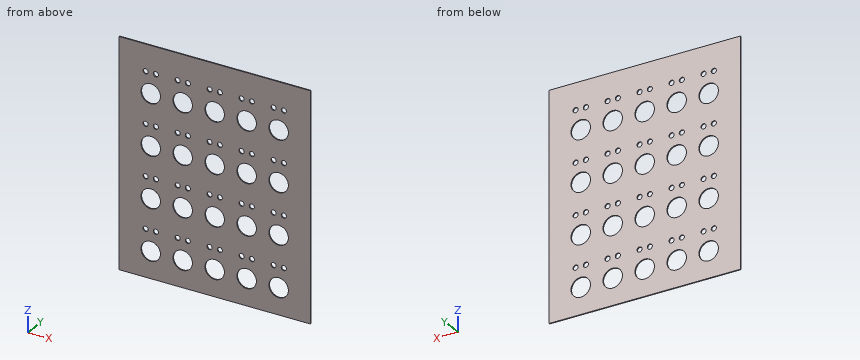
```python
from build123d import *

# Parameters (mm, degrees)
SKETCH1_W           = 187
SKETCH1_H           = 222
SKETCH1_R           = 2.5
SKETCH1_R_2         = 9.5
BOSS_EXTRUDE1_DEPTH = 1


with BuildPart() as part:
    # Sketch1 → Boss-Extrude1 (new body)
    with BuildSketch(Plane(origin=(0, 0, 0), x_dir=(1, 0, 0), z_dir=(0, 1, 0))):
        with Locations((64.462554676, 36.018217652)):
            Rectangle(SKETCH1_W, SKETCH1_H)
        with Locations((-3.037445324, -48.981782348)):
            Circle(SKETCH1_R, mode=Mode.SUBTRACT)
        with Locations((6.962554676, -48.981782348)):
            Circle(SKETCH1_R, mode=Mode.SUBTRACT)
        with Locations((28.212554676, -48.981782348)):
            Circle(SKETCH1_R, mode=Mode.SUBTRACT)
        with Locations((38.212554676, -48.981782348)):
            Circle(SKETCH1_R, mode=Mode.SUBTRACT)
        with Locations((1.962554676, -28.981782348)):
            Circle(SKETCH1_R_2, mode=Mode.SUBTRACT)
        with Locations((33.212554676, -28.981782348)):
            Circle(SKETCH1_R_2, mode=Mode.SUBTRACT)
        with Locations((59.462554676, -48.981782348)):
            Circle(SKETCH1_R, mode=Mode.SUBTRACT)
        with Locations((69.462554676, -48.981782348)):
            Circle(SKETCH1_R, mode=Mode.SUBTRACT)
        with Locations((64.462554676, -28.981782348)):
            Circle(SKETCH1_R_2, mode=Mode.SUBTRACT)
        with Locations((90.712554676, -48.981782348)):
            Circle(SKETCH1_R, mode=Mode.SUBTRACT)
        with Locations((100.712554676, -48.981782348)):
            Circle(SKETCH1_R, mode=Mode.SUBTRACT)
        with Locations((95.712554676, -28.981782348)):
            Circle(SKETCH1_R_2, mode=Mode.SUBTRACT)
        with Locations((121.962554676, -48.981782348)):
            Circle(SKETCH1_R, mode=Mode.SUBTRACT)
        with Locations((131.962554676, -48.981782348)):
            Circle(SKETCH1_R, mode=Mode.SUBTRACT)
        with Locations((126.962554676, -28.981782348)):
            Circle(SKETCH1_R_2, mode=Mode.SUBTRACT)
        with Locations((-3.037445324, 1.018217652)):
            Circle(SKETCH1_R, mode=Mode.SUBTRACT)
        with Locations((6.962554676, 1.018217652)):
            Circle(SKETCH1_R, mode=Mode.SUBTRACT)
        with Locations((1.962554676, 21.018217652)):
            Circle(SKETCH1_R_2, mode=Mode.SUBTRACT)
        with Locations((28.212554676, 1.018217652)):
            Circle(SKETCH1_R, mode=Mode.SUBTRACT)
        with Locations((38.212554676, 1.018217652)):
            Circle(SKETCH1_R, mode=Mode.SUBTRACT)
        with Locations((33.212554676, 21.018217652)):
            Circle(SKETCH1_R_2, mode=Mode.SUBTRACT)
        with Locations((59.462554676, 1.018217652)):
            Circle(SKETCH1_R, mode=Mode.SUBTRACT)
        with Locations((69.462554676, 1.018217652)):
            Circle(SKETCH1_R, mode=Mode.SUBTRACT)
        with Locations((64.462554676, 21.018217652)):
            Circle(SKETCH1_R_2, mode=Mode.SUBTRACT)
        with Locations((90.712554676, 1.018217652)):
            Circle(SKETCH1_R, mode=Mode.SUBTRACT)
        with Locations((100.712554676, 1.018217652)):
            Circle(SKETCH1_R, mode=Mode.SUBTRACT)
        with Locations((95.712554676, 21.018217652)):
            Circle(SKETCH1_R_2, mode=Mode.SUBTRACT)
        with Locations((121.962554676, 1.018217652)):
            Circle(SKETCH1_R, mode=Mode.SUBTRACT)
        with Locations((131.962554676, 1.018217652)):
            Circle(SKETCH1_R, mode=Mode.SUBTRACT)
        with Locations((126.962554676, 21.018217652)):
            Circle(SKETCH1_R_2, mode=Mode.SUBTRACT)
        with Locations((-3.037445324, 51.018217652)):
            Circle(SKETCH1_R, mode=Mode.SUBTRACT)
        with Locations((6.962554676, 51.018217652)):
            Circle(SKETCH1_R, mode=Mode.SUBTRACT)
        with Locations((1.962554676, 71.018217652)):
            Circle(SKETCH1_R_2, mode=Mode.SUBTRACT)
        with Locations((28.212554676, 51.018217652)):
            Circle(SKETCH1_R, mode=Mode.SUBTRACT)
        with Locations((38.212554676, 51.018217652)):
            Circle(SKETCH1_R, mode=Mode.SUBTRACT)
        with Locations((33.212554676, 71.018217652)):
            Circle(SKETCH1_R_2, mode=Mode.SUBTRACT)
        with Locations((59.462554676, 51.018217652)):
            Circle(SKETCH1_R, mode=Mode.SUBTRACT)
        with Locations((69.462554676, 51.018217652)):
            Circle(SKETCH1_R, mode=Mode.SUBTRACT)
        with Locations((64.462554676, 71.018217652)):
            Circle(SKETCH1_R_2, mode=Mode.SUBTRACT)
        with Locations((90.712554676, 51.018217652)):
            Circle(SKETCH1_R, mode=Mode.SUBTRACT)
        with Locations((100.712554676, 51.018217652)):
            Circle(SKETCH1_R, mode=Mode.SUBTRACT)
        with Locations((95.712554676, 71.018217652)):
            Circle(SKETCH1_R_2, mode=Mode.SUBTRACT)
        with Locations((121.962554676, 51.018217652)):
            Circle(SKETCH1_R, mode=Mode.SUBTRACT)
        with Locations((131.962554676, 51.018217652)):
            Circle(SKETCH1_R, mode=Mode.SUBTRACT)
        with Locations((126.962554676, 71.018217652)):
            Circle(SKETCH1_R_2, mode=Mode.SUBTRACT)
        with Locations((-3.037445324, 101.018217652)):
            Circle(SKETCH1_R, mode=Mode.SUBTRACT)
        with Locations((6.962554676, 101.018217652)):
            Circle(SKETCH1_R, mode=Mode.SUBTRACT)
        with Locations((1.962554676, 121.018217652)):
            Circle(SKETCH1_R_2, mode=Mode.SUBTRACT)
        with Locations((28.212554676, 101.018217652)):
            Circle(SKETCH1_R, mode=Mode.SUBTRACT)
        with Locations((38.212554676, 101.018217652)):
            Circle(SKETCH1_R, mode=Mode.SUBTRACT)
        with Locations((33.212554676, 121.018217652)):
            Circle(SKETCH1_R_2, mode=Mode.SUBTRACT)
        with Locations((59.462554676, 101.018217652)):
            Circle(SKETCH1_R, mode=Mode.SUBTRACT)
        with Locations((69.462554676, 101.018217652)):
            Circle(SKETCH1_R, mode=Mode.SUBTRACT)
        with Locations((64.462554676, 121.018217652)):
            Circle(SKETCH1_R_2, mode=Mode.SUBTRACT)
        with Locations((90.712554676, 101.018217652)):
            Circle(SKETCH1_R, mode=Mode.SUBTRACT)
        with Locations((100.712554676, 101.018217652)):
            Circle(SKETCH1_R, mode=Mode.SUBTRACT)
        with Locations((95.712554676, 121.018217652)):
            Circle(SKETCH1_R_2, mode=Mode.SUBTRACT)
        with Locations((121.962554676, 101.018217652)):
            Circle(SKETCH1_R, mode=Mode.SUBTRACT)
        with Locations((131.962554676, 101.018217652)):
            Circle(SKETCH1_R, mode=Mode.SUBTRACT)
        with Locations((126.962554676, 121.018217652)):
            Circle(SKETCH1_R_2, mode=Mode.SUBTRACT)
    extrude(amount=BOSS_EXTRUDE1_DEPTH)


solid = part.part
```
For this review, take the finished solid that the model builds, in its own axes (mm). Round coordinates to 2 decimals unless told otherwise and drop trailing zeros. Use one line per item in the form item = value.
1) Clearance check with a flat-ended pin moving along its axis: pin 1 (4 mm diameter, centred on x = 69.46, z = -1.02, fed in from -Y). State where the tip first meets the part, or that it passes through.
Found:
pin_1 = through
2) To check wall thickness, follow L1, parallel to X at y = 0.15, z = -68; L2, parallel to X at y = 0.35, z = -69; L3, parallel to Z at x = 25.5, y = 0.8. State the ranges of each line that lie inside material, in increasing order. Write a range as from..to.
Found:
L1 = -29.04..-7.05, 10.97..24.2, 42.22..55.45, 73.47..86.7, 104.72..117.95, 135.97..157.96
L2 = -29.04..-7.32, 11.25..23.93, 42.5..55.18, 73.75..86.43, 105..117.68, 136.25..157.96
L3 = -147.02..-126.56, -115.47..-76.56, -65.47..-26.56, -15.47..23.44, 34.53..74.98
3) Take a section at A-A, the plane y = 0.2. Count the separate pieces of the cut face and the enclosed holes in it, and give its area (3 significant figures).
Found:
separate_pieces = 1
enclosed_holes = 60
area = 35,100 mm2
